Autodesk Inventor part; units mm, degrees
ref_plane "YZ Plane" through (0, 0, 0) normal (1, 0, 0) x (0, 1, 0)
ref_plane "XZ Plane" through (0, 0, 0) normal (0, 1, 0) x (-1, 0, 0)
ref_plane "XY Plane" through (0, 0, 0) normal (0, 0, 1) x (1, 0, 0)
sketch "Sketch1" plane through (0, 0, 0) normal (0, 0, 1) x (1, 0, 0)
  line L0 (0, 0) -> (-178.9061, 0)
  line L1 (-178.9061, 0) -> (-178.9061, -1490)
  line L2 (-178.9061, -1490) -> (0, -1490)
  line L3 (0, -1490) -> (0, 0)
  line L4 (-178.9061, -1390) -> (-66, -1390)
  line L5 (-66, -1390) -> (-66, -1385)
  line L6 (-66, -1385) -> (-178.9061, -1385)
  line L7 (-178.9061, -1385) -> (-178.9061, -1390)
  line L8 (-178.9061, -890) -> (-66, -890)
  line L9 (-66, -890) -> (-66, -885)
  line L10 (-66, -885) -> (-178.9061, -885)
  line L11 (-178.9061, -885) -> (-178.9061, -890)
  line L12 (-178.9061, -390) -> (-66, -390)
  line L13 (-66, -390) -> (-66, -385)
  line L14 (-66, -385) -> (-178.9061, -385)
  line L15 (-178.9061, -385) -> (-178.9061, -390)
  circle A0 centre (-178.9061, -155) radius 30
  point P0 (-178.9061, -390)
  point P1 (-178.9061, -885)
  point P2 (-178.9061, -125)
  point P3 (-178.9061, -185)
  dimension "d0" = 1490
  dimension "d1" = 178.9061
  dimension "d2" = 5
  dimension "d4" = 100
  dimension "d7" = 500
  dimension "d23" = 66
  dimension "d28" = 60
  dimension "d30" = 1335
extrude "Plate1" add sketch "Sketch1" along normal blind 4 contours L3 L2 L1 L4 L5 L6 L8 L9 L10 L12 L13 L14 A0 L0
sketch "Sketch2" plane through (-4, 0, 0) normal (1, 0, 0) x (0, 1, 0)
  line L0 (-1490, 0) -> (0, 0)
  line L1 (0, 0) -> (0, 60)
  line L2 (0, 60) -> (-1490, 60)
  line L3 (-1490, 60) -> (-1490, 0)
edge flange "Flange1" height 60 angle 90 thickness 4 bend radius 4 thickness toward (1, 0, 0) relief tear relief width 4 relief depth 2 edges at (0, -745, 4) wall of the first edge with corners at (-4, -1490, 0) (-4, 0, 0) (-4, 0, 60) (-4, -1490, 60)
bend "Bend1"
corner "Corner1"
chamfer "Corner Chamfer1" distance 3 angle 45 6 edges at (-178.9061, -1390, 2) (-178.9061, -1385, 2) (-178.9061, -890, 2) (-178.9061, -885, 2) (-178.9061, -385, 2) (-178.9061, -390, 2)
equation "\"d0\" = Стрингер_длина"
equation "\"d1\" = стрингер_глубина_2"
equation "\"d2\" = паз_под_стрингер_толщина"
equation "\"d23\" = паз_под_стрингер_глубина - Thickness"
equation "\"d28\" = 2 * радиус_выреза_под_сварку"
equation "\"d12\" = Thickness"
equation "\"d13\" = BendReliefWidth"
equation "\"d14\" = BendReliefDepth"
equation "\"d15\" = MinimumRemnant"
equation "\"d16\" = TransitionRadius"
equation "\"d17\" = ребро_усилителей"
equation "\"d19\" = BendRadius"
equation "\"d20\" = CornerReliefSize"
equation "\"d21\" = GapSize"
equation "\"d22\" = JacobiRadiusSize"
equation "\"BendRadius\" = Thickness"
equation "\"BendReliefWidth\" = Thickness"
equation "\"BendReliefDepth\" = 0.5 * Thickness"
equation "\"CornerReliefSize\" = 4 * Thickness"
equation "\"MinimumRemnant\" = 2 * Thickness"
equation "\"TransitionRadius\" = BendRadius"
equation "\"JacobiRadiusSize\" = BendRadius"
equation "\"GapSize\" = Thickness"
properties part number "0235 GBK stringer 2" material "Steel"
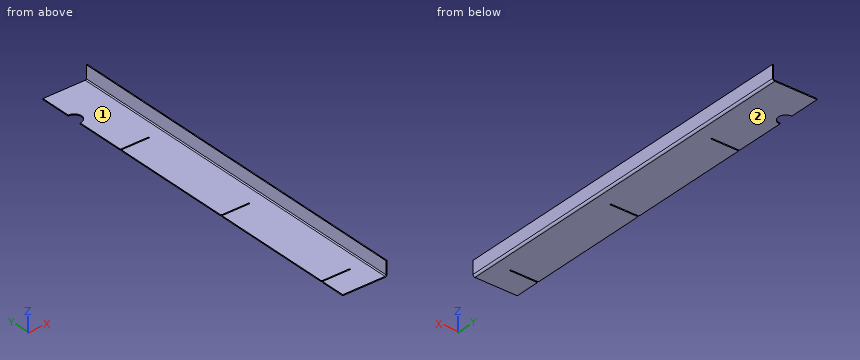
Design review of the part built by this model. Coordinates are the model's own, in mm. Face numbers are marked on the shaded views. A direction names the side the tool comes from. Give positions to 0.01 mm unless a question says otherwise; leave off trailing zeros. Order: outer loops, then holes, each group sorted by start corner. A loop starts at its lowest first (then second) coordinate and runs counter-clockwise, first axis right, second up. Notation, with made-up numbers: (13.25, 47) -> (55.25, 47) arc R33 cw to (55.25, 82) -> close; hole circle Ø2 at (62.25, 64.25). An arc over 180 degrees is marked (long way). Write item = value, one per line. Start each with the question number.
(1) To check wall thickness, follow line 1 along Z through (x, y) = (-45.5, -939.5); line 2 along X through (y, z) = (-1420, 56); line 3 along X through (y, z) = (-1043, 6.5). State the ranges of each line that lie inside material, in increasing order.
(2) We need section B-B on y = -962. Write out the cut boundary in (x, z), plus the area to 3 significant figures.
(3) For the marked faces 1 and 2, list the 3-axis set-ups (+Z, -Z, +X, -X, +Y, -Y) from which the entire face can be reached by the end or side of a thin tool; tool diameter is ignored.
(4) We need section A-A on x = -97. Write out the cut boundary in (y, z), plus the area to 3 significant figures.
(5) For pin 1 (4 mm diameter, centred on y = -1126, z = 12.5, fed in from -X); pin 2 (1 mm diameter, centred on x = -114.5, y = -1070.5, fed in from +Z); pin 3 (2 mm diameter, centred on y = -886.5, z = 1.5, fed in from -X), all flat-tipped, find the tip position at first contact; note any pin that passes through.
(6) We need section D-D on y = -155. Write out the cut boundary in (x, z), plus the area to 3 significant figures.
(7) We need section C-C on x = -163.5. Write out the cut boundary in (y, z), plus the area to 3 significant figures.
Numbers:
q1.line_1 = 0 to 4
q1.line_2 = -4 to 0
q1.line_3 = -4.29 to -0.14
q2.outline = (-178.91, 0) -> (-8, 0) arc R8 ccw to (0, 8) -> (0, 60) -> (-4, 60) -> (-4, 8) arc R4 cw to (-8, 4) -> (-178.91, 4) -> close
q2.area = 929 mm^2
q3.face_1 = +Z, -X, +Y, -Y
q3.face_2 = -Z, +X, -X, +Y, -Y
q4.outline = (-1490, 0) -> (-1390, 0) -> (-1390, 4) -> (-1490, 4) -> close; (-1385, 0) -> (-890, 0) -> (-890, 4) -> (-1385, 4) -> close; (-885, 0) -> (-390, 0) -> (-390, 4) -> (-885, 4) -> close; (-385, 0) -> (0, 0) -> (0, 4) -> (-385, 4) -> close
q4.area = 5,900 mm^2
q5.pin_1 = -4
q5.pin_2 = 4
q5.pin_3 = -66
q6.outline = (-148.91, 0) -> (-8, 0) arc R8 ccw to (0, 8) -> (0, 60) -> (-4, 60) -> (-4, 8) arc R4 cw to (-8, 4) -> (-148.91, 4) -> close
q6.area = 809 mm^2
q7.outline = (-1490, 0) -> (-1390, 0) -> (-1390, 4) -> (-1490, 4) -> close; (-1385, 0) -> (-890, 0) -> (-890, 4) -> (-1385, 4) -> close; (-885, 0) -> (-390, 0) -> (-390, 4) -> (-885, 4) -> close; (-385, 0) -> (-180.74, 0) -> (-180.74, 4) -> (-385, 4) -> close; (-129.26, 0) -> (0, 0) -> (0, 4) -> (-129.26, 4) -> close
q7.area = 5,690 mm^2
